from build123d import *

# Parameters (mm, degrees)
SKETCH_1_W      = 15
SKETCH_1_H      = 99
EXTRUDE_1_DEPTH = 2
EXTRUDE_2_DEPTH = 5
EXTRUDE_3_DEPTH = 5


with BuildPart() as part:
    # 草图1 → 凸台-拉伸1 (new body)
    with BuildSketch(Plane(origin=(0, 0, 0), x_dir=(1, 0, 0), z_dir=(0, 1, 0))):
        with Locations((-2.772511848, -40.347156398)):
            Rectangle(SKETCH_1_W, SKETCH_1_H)
    extrude(amount=EXTRUDE_1_DEPTH)

    # 草图3 → 凸台-拉伸2 (add)
    with BuildSketch(Plane.XY):
        Polygon((-4.810549778, 0), (4.727488152, -5.543936954), (4.727488152, -4.491111673), (-2.999221917, 0), align=None)
    extrude(amount=EXTRUDE_2_DEPTH)

    # 草图5 → 凸台-拉伸3 (add)
    with BuildSketch(Plane.XY.offset(80)):
        Polygon((-4.810549778, 0), (4.727488152, -5.543936954), (4.727488152, -4.491111673), (-2.999221917, 0), align=None)
    extrude(amount=EXTRUDE_3_DEPTH)


solid = part.part
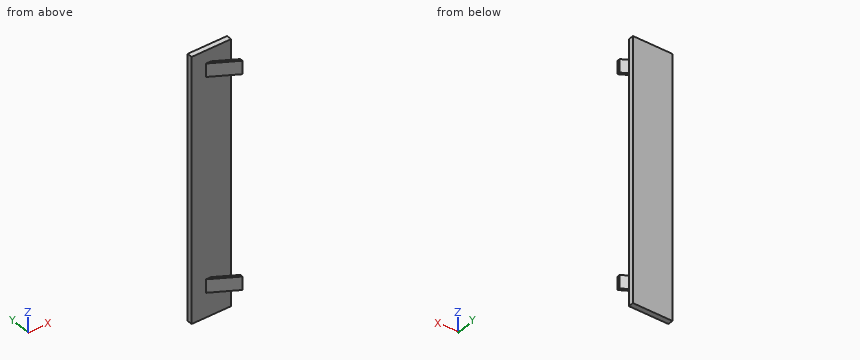
The listing builds one solid part. Answer for the finished solid, in the listing's coordinates (mm). Coordinates: 2 decimals unless noted, no trailing zeros. Write each loop counter-clockwise with the first axis right and the second up, starting at its lowest first coordinate (ties: lowest second). Pieces come first, ordered by that corner, then holes. Notation, with made-up numbers: (69, 15) - (126, 15) arc R19 cw to (126, 19) - close; hole circle Ø9 at (83.5, 30.25). An arc over 180 degrees is marked (long way). Put each result on its own line as item: value.
1. Flat-ended cylindrical pins translate along their axes: pin 1 Ø1 at (x, z) = (-1, 21.5) entering from -Y; pin 2 Ø1.7 at (x, y) = (2, -3) entering from +Z. Find the tip coordinate at first contact, or state that the pin passes through.
Answer sheet:
pin 1: stops at y = 0
pin 2: stops at z = 85
2. The part is cut by section B-B on y = -2.5. Give the vertices of the cut face in (x, z).
Answer sheet:
outline: (-0.51, 0) - (1.3, 0) - (1.3, 5) - (-0.51, 5) - close; (-0.51, 80) - (1.3, 80) - (1.3, 85) - (-0.51, 85) - close
3. The part is cut by section C-C on z = 31.5. Give the vertices of the cut face in (x, y), plus the area to 3 significant figures.
Answer sheet:
outline: (-10.27, 0) - (4.73, 0) - (4.73, 2) - (-10.27, 2) - close
area: 30.0 mm^2
4. The part is cut by section D-D on x = -9. Give the vertices of the cut face in (y, z), plus the area to 3 significant figures.
Answer sheet:
outline: (0, -9.15) - (2, -9.15) - (2, 89.85) - (0, 89.85) - close
area: 198 mm^2
5. Find the intervals of material crossed by line 1 along Z through (x, y) = (3.5, -4); line 2 along Y through (x, z) = (-6.5, 47); line 3 along Y through (x, z) = (0.5, 2.5), in increasing order. Write a range as from..to.
Answer sheet:
line 1: z = 0..5, 80..85
line 2: y = 0..2
line 3: y = -3.09..-2.03, 0..2
6. The part is cut by section A-A on x = -1. Give the vertices of the cut face in (y, z).
Answer sheet:
outline: (-2.21, 0) - (-1.16, 0) - (-1.16, 5) - (-2.21, 5) - close; (-2.21, 80) - (-1.16, 80) - (-1.16, 85) - (-2.21, 85) - close; (0, -9.15) - (2, -9.15) - (2, 89.85) - (0, 89.85) - close
